Geometry: final body of the model. Coordinates: model frame, mm. Give positions to 0.01 mm unless a question says otherwise; leave off trailing zeros. Order: outer loops, then holes, each group sorted by start corner. A loop starts at its lowest first (then second) coordinate and runs counter-clockwise, first axis right, second up. Notation, with made-up numbers: M 30.25,15 L 36.25,15 A20 ccw 36.25,46 Z; hole C -35.5,-7.75 d1. An arc over 180 degrees is marked long. Use CSV: the item, a comma, the result in double quotes.
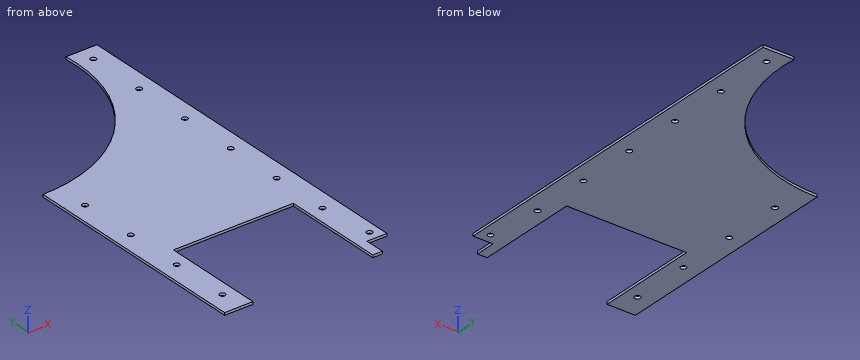
Autodesk Inventor part; units mm, degrees
ref_plane "YZ Plane" through (0, 0, 0) normal (1, 0, 0) x (0, 1, 0)
ref_plane "XZ Plane" through (0, 0, 0) normal (0, 1, 0) x (-1, 0, 0)
ref_plane "XY Plane" through (0, 0, 0) normal (0, 0, 1) x (1, 0, 0)
sketch "Sketch1" plane through (0, 0, 0) normal (0, 0, 1) x (1, 0, 0)
  line L0 (229.6952, -414.7737) -> (228.902, -414.7737)
  line L1 (202.9458, -491.49) -> (202.9458, -465.836)
  line L2 (202.9458, -465.836) -> (228.5998, -465.836)
  line L3 (202.9458, -491.49) -> (-0.0002, -491.49)
  line L4 (-0.0002, -491.49) -> (-0.0002, -189.4332)
  arc A0 (-0.0002, -189.4332) -> (188.7124, 16.51) centre (0, 0) ccw
  line L5 (0, 0) -> (188.7124, 16.51) construction
  line L6 (0, 0) -> (-0.0002, -189.4332) construction
  line L7 (228.5998, -465.836) -> (228.5998, 16.51)
  line L8 (228.5998, 16.51) -> (188.7124, 16.51)
  circle A1 centre (20.5738, -232.664) radius 3.5687
  circle A2 centre (20.5738, -308.864) radius 3.5687
  circle A3 centre (20.5738, -385.064) radius 3.5687
  circle A4 centre (20.5738, -461.264) radius 3.5687
  circle A5 centre (215.8998, -453.136) radius 3.5687
  circle A6 centre (208.0258, -385.064) radius 3.5687
  circle A7 centre (208.0258, -308.864) radius 3.5687
  circle A8 centre (208.0258, -232.664) radius 3.5687
  circle A9 centre (208.0301, -156.464) radius 3.5687
  circle A10 centre (208.0258, -80.264) radius 3.5687
  circle A11 centre (208.0258, -4.064) radius 3.5687
  line L9 (36.3726, -491.49) -> (190.4998, -491.49)
  line L10 (190.4998, -491.49) -> (190.4998, -359.41)
  line L11 (190.4998, -359.41) -> (36.3726, -359.41)
  line L12 (36.3726, -359.41) -> (36.3726, -491.49)
  point P0 (208.0258, -461.264)
  dimension "d15" = 25.654
  dimension "d59" = 95
  dimension "d60" = 189.4332
  dimension "d61" = 508
  dimension "d62" = 76.2
  dimension "d63" = 76.2
  dimension "d65" = 20.5697
  dimension "d66" = 20.574
  dimension "d67" = 20.574
  dimension "d68" = 76.2
  dimension "d69" = 76.2
  dimension "d70" = 76.2
  dimension "d71" = 76.2
  dimension "d73" = 25.654
  dimension "d74" = 12.7
  dimension "d75" = 76.2
  dimension "d76" = 76.2
  dimension "d77" = 76.2
  dimension "d78" = 43.2308
  dimension "d79" = 20.574
  dimension "d80" = 20.574
  dimension "d81" = 20.574
  dimension "d82" = 20.574
  dimension "d85" = 7.1374
  dimension "d86" = 7.1374
  dimension "d87" = 7.1374
  dimension "d88" = 7.1374
  dimension "d89" = 7.1374
  dimension "d91" = 7.1374
  dimension "d92" = 7.1374
  dimension "d93" = 7.1374
  dimension "d94" = 7.1374
  dimension "d95" = 7.1374
  dimension "d96" = 7.1374
  dimension "d99" = 228.6
  dimension "d100" = 12.7
  dimension "d103" = 20.574
  dimension "d104" = 20.574
  dimension "d105" = 20.574
  dimension "d106" = 20.574
  dimension "d108" = 30.226
  dimension "d109" = 106.426
  dimension "d112" = 154.1272
  dimension "d113" = 132.08
  dimension "d114" = 12.446
extrude "Extrusion6" add sketch "Sketch1" along normal blind 3.175 contours L3 L10 L11 L12 L4 A0 L8 L7 L2 L1
properties part number "LauncherSidePlateRev2"
1. Section B-B, the plane z = 1.8. Give the number of separate pieces and of enclosed holes in the cut face, plus the area to 3 significant figures.
Answer:
separate pieces,"1"
enclosed holes,"11"
area,"63,400 mm2"
2. Section C-C, the plane x = 171.5. Return the cut outline in (y, z) (3 decimals), plus the area to 3 significant figures.
Answer:
outline,"M -359.41,0 L -80.453,0 L -80.453,3.175 L -359.41,3.175 Z"
area,"886 mm2"
3. Section D-D, the plane y = -118. Return the cut outline in (x, z) (3 decimals).
Answer:
outline,"M 148.192,0 L 228.6,0 L 228.6,3.175 L 148.192,3.175 Z"
4. Line query: line 1 (X direction, y = -380.5, z = 0.9); line 2 (Y direction, x = 17.5, z = 0.9); line 3 (X direction, y = -462.5, z = 1.2). Output: solid intervals per line, ascending.
Answer:
line 1,"0 to 36.37, 190.5 to 228.6"
line 2,"-491.49 to -463.08, -459.45 to -386.88, -383.25 to -310.68, -307.05 to -234.48, -230.85 to -188.62"
line 3,"0 to 17.23, 23.92 to 36.37, 190.5 to 228.6"
5. Section A-A, the plane y = -408.5. Return the cut outline in (x, z) (3 decimals).
Answer:
outline,"M 0,0 L 36.373,0 L 36.373,3.175 L 0,3.175 Z; M 190.5,0 L 228.6,0 L 228.6,3.175 L 190.5,3.175 Z"
6. Pin query (flat end, axial travel): pin 1 Ø9.5 at (x, y) = (208.03, -80.26) entering from +Z (3 decimals); pin 2 Ø4.5 at (x, y) = (215.9, -453.14) entering from +Z; pin 3 Ø1.6 at (x, z) = (216, 1) entering from -Y; pin 4 Ø1.5 at (x, z) = (32, 2) entering from +Y. Return the tip coordinate at first contact, or that it passes through.
Answer:
pin 1,"z = 3.175"
pin 2,"through"
pin 3,"y = -465.84"
pin 4,"y = -186.58"
